Can you work these out from the model? Positions are in its coordinate system, mm. A direction names the side the tool comes from. Round coordinates to 2 decimals unless told otherwise and drop trailing zeros. Order: outer loops, then holes, each group sorted by start corner. A loop starts at its lowest first (then second) coordinate and runs counter-clockwise, first axis right, second up.
Autodesk Inventor part; units mm, degrees
ref_plane "YZ Plane" through (0, 0, 0) normal (1, 0, 0) x (0, 1, 0)
ref_plane "XZ Plane" through (0, 0, 0) normal (0, 1, 0) x (-1, 0, 0)
ref_plane "XY Plane" through (0, 0, 0) normal (0, 0, 1) x (1, 0, 0)
sketch "Sketch1" plane through (0, 0, 0) normal (0, 1, 0) x (-1, 0, 0)
  line L0 (-20, 12.5) -> (20, 12.5)
  line L1 (20, 12.5) -> (20, -12.5)
  line L2 (20, -12.5) -> (-20, -12.5)
  line L3 (-20, -12.5) -> (-20, 12.5)
  line L4 (-20, 12.5) -> (20, -12.5) construction
  line L5 (20, 12.5) -> (-20, -12.5) construction
  circle A0 centre (-4, 8.75) radius 2.25
  circle A1 centre (-4.5, -8.75) radius 2.25
  point P0 (0, 0)
  dimension "d0" = 40
  dimension "d1" = 25
  dimension "d49" = 4.5
  dimension "d50" = 4.5
extrude "Extrusion1" add sketch "Sketch1" along normal blind 3 contours L0 L1 L2 L3 | A0 | A1
sketch "Sketch3" plane through (-20, 0, -12.5) normal (-1, 0, 0) x (0, 0, 1)
  line L0 (0, 0) -> (25, 0)
  line L1 (0, 0) -> (25, 0)
  line L2 (25, 0) -> (25, 22)
  line L3 (25, 22) -> (0, 22)
  line L4 (0, 22) -> (0, 0)
  point P0 (12.5, 0)
  dimension "d14" = 22
extrude "Extrusion4" add sketch "Sketch3" along normal blind 9
sketch "Sketch4" plane through (-20, 22, 12.5) normal (0, 1, 0) x (1, 0, 0)
  line L0 (-4.7075, 24) -> (-1.5075, 24)
  line L1 (-1.5075, 24) -> (-1.5075, 1)
  line L2 (-1.5075, 1) -> (-4.7075, 1)
  line L3 (-4.7075, 1) -> (-4.7075, 24)
  point P0 (20, 12.5)
  dimension "d17" = 3.2
  dimension "d18" = 23
extrude "Extrusion5" cut sketch "Sketch4" against normal blind 21
sketch "Sketch6" plane through (-21.5075, 22, -11.5) normal (-1, 0, 0) x (0, 0, 1)
  line L0 (0, 0) -> (23, 0)
  line L1 (0, 0) -> (23, 0)
  line L2 (23, 0) -> (23, -3)
  line L3 (23, -3) -> (0, -3)
  line L4 (0, -3) -> (0, 0)
  point P0 (11.5, -22)
  dimension "d26" = 3
extrude "Extrusion7" cut sketch "Sketch6" against normal blind 3
sketch "Sketch5" plane through (-29, 0, -12.5) normal (-1, 0, 0) x (0, 0, 1)
  line L0 (20, 18.5) -> (20, 3.5)
  line L1 (20, 3.5) -> (5, 3.5)
  line L2 (5, 3.5) -> (5, 18.5)
  line L3 (5, 18.5) -> (20, 18.5)
  point P0 (12.5, 0)
  dimension "d21" = 15
  dimension "d22" = 15
extrude "Extrusion6" cut sketch "Sketch5" against normal blind 7
sketch "Sketch7" plane through (-29, 0, -12.5) normal (-1, 0, 0) x (0, 0, 1)
  line L0 (20, 3.5) -> (5, 3.5)
  line L1 (5, 3.5) -> (2, 3.5)
  line L2 (2, 3.5) -> (2, 22.5)
  line L3 (2, 22.5) -> (5, 22.5)
  line L4 (5, 22.5) -> (5, 3.5)
  line L5 (5, 22.5) -> (20, 22.5)
  line L6 (20, 22.5) -> (20, 18.5)
  line L7 (20, 18.5) -> (5, 18.5)
  line L8 (5, 18.5) -> (5, 22.5)
  line L9 (20, 3.5) -> (20, 22.5)
  line L10 (20, 22.5) -> (23, 22.5)
  line L11 (23, 22.5) -> (23, 3.5)
  line L12 (23, 3.5) -> (20, 3.5)
  line L13 (25, 0) -> (25, 22)
  point P0 (12.5, 0)
  dimension "d29" = 3
  dimension "d30" = 19
  dimension "d31" = 15
  dimension "d32" = 3
extrude "Extrusion8" add sketch "Sketch7" along normal blind 1 contours L1 L2 L3 L4
extrude "Extrusion9" add sketch "Sketch7" along normal blind 22 contours L9 L6 L10 L11 L12 | L7 L4 L5 L6
extrude "Extrusion10" add sketch "Sketch7" along normal blind 22 contours L1 L2 L3 L4
sketch "Sketch8" plane through (20, 0, 12.5) normal (0, 0, 1) x (1, 0, 0)
  line L0 (-40, 22) -> (-49, 22)
  line L1 (-49, 22) -> (-40, 22)
  line L2 (-40, 22) -> (-40, 0)
  line L3 (-40, 0) -> (-49, 0)
  line L4 (-49, 0) -> (-49, 22)
  point P0 (-20, 0)
extrude "Extrusion11" add sketch "Sketch8" along normal blind 2
sketch "Sketch9" plane through (20, 0, -12.5) normal (0, 0, -1) x (-1, 0, 0)
  line L0 (40, 22) -> (44.7075, 22)
  line L1 (49, 22) -> (40, 22)
  line L2 (40, 22) -> (40, 0)
  line L3 (40, 0) -> (49, 0)
  line L4 (49, 0) -> (49, 22)
  point P0 (20, 0)
extrude "Extrusion12" add sketch "Sketch9" along normal blind 2
sketch "Sketch10" plane through (-20, 0, -12.5) normal (1, 0, 0) x (0, 0, -1)
  line L0 (-27, 0) -> (-27, 22)
  line L1 (2, 22) -> (2, 0)
  line L2 (-27, 22) -> (2, 22)
  line L3 (2, 22) -> (2, 0)
  line L4 (2, 0) -> (-27, 0)
  line L5 (-27, 0) -> (-27, 22)
  point P0 (-12.5, 0)
extrude "Extrusion13" add sketch "Sketch10" along normal blind 2
sketch "Sketch11" plane through (-20, 0, -12.5) normal (-1, 0, 0) x (0, 0, 1)
  line L0 (1, 22) -> (1, 19)
  line L1 (1, 22) -> (24, 22)
  line L2 (1, 19) -> (1, 22)
  line L3 (1, 22) -> (24, 22)
  line L4 (24, 22) -> (24, 19)
  line L5 (24, 19) -> (1, 19)
  point P0 (12.5, 0)
extrude "Extrusion14" cut sketch "Sketch11" against normal blind 2
extrude "Extrusion15" cut sketch "Sketch1" along normal blind 3 contours A0 | A1
fillet "Fillet2" radius 3 2 edges at (-40, 22.5, 10.5) (-40, 22.5, -10.5)
sketch "Sketch12" plane through (20, 0, -12.5) normal (0, 0, -1) x (-1, 0, 0)
  line L0 (0, 3) -> (38, 3)
  line L1 (0, 3) -> (10, 3)
  line L2 (10, 3) -> (10, 0)
  line L3 (10, 0) -> (0, 0)
  line L4 (0, 0) -> (0, 3)
  point P0 (20, 0)
  dimension "d54" = 10
extrude "Extrusion16" cut sketch "Sketch12" against normal blind 25
properties part number "rgb-mount-group2"
(1) I want a section at B-B, the plane x = 4. List the corners of the cut face in (y, z) for me, plus the area to 3 significant figures.
(2) I want a section at C-C, the plane y = 6.25. List the corners of the cut face in (x, z) for me.
(3) On a 3-axis mill with a long thin cutter (end or side, diameter ignored), from which of +Z, -Z, +X, -X, +Y, -Y can I reach the whole of each face in a straight line? I mean faces 1 (the face through (-38, 11, -7.5)), 2 (the face through (-26, 22, 0)), 3 (the face through (-20, 19, 0)), 4 (the face through (-40, 12, 10.5)), 5 (the face through (-39.85, 21.64, 9.6)). Say none if no direction works.
(4) I'm going to push flat-ended pins straight in: pin 1 Ø4.5 at (x, y) = (-43.5, 10.5) entering from -Z; pin 2 Ø8 at (x, z) = (-40, 6.5) entering from -Y; pin 3 Ø3 at (x, z) = (-19.5, 1.5) entering from +Y; pin 4 Ø4.5 at (x, z) = (-27, -1.5) entering from +Y. Where does each tip first touch, or does it pass through?
(5) Please list where these lines run through material, in increasing order: probe 1 along Z at (x, y) = (-27.5, 7); probe 2 along X at (y, z) = (3.25, 6.75); probe 3 along Z at (x, y) = (4, 2.05).
(6) I want a section at A-A, the plane z = -2.25. List the corners of the cut face in (x, y) for me.
(7) I want a section at D-D, the plane x = -6.5. List the corners of the cut face in (y, z) for me, plus the area to 3 significant figures.
(8) If we mould it in two halves opening along Z, with no side actions, what happens to faces 6 (the face through (-40, 11, -10.5)), 7 (the face through (-27, 3.5, 0)), 8 (the face through (-51, 19, 0))? For each: pulls with the +Z half, pulls with the -Z half, needs draft (parallel to the pull), parting line crosses it, or undercut.
Ans:
1. outline: (0, -12.5) - (3, -12.5) - (3, -10.94) - (0, -10.94) - close; (0, -6.56) - (3, -6.56) - (3, 6.5) - (0, 6.5) - close; (0, 11) - (3, 11) - (3, 12.5) - (0, 12.5) - close
1. area: 48.3 mm2
2. outline: (-51, -10.5) - (-29, -10.5) - (-29, -14.5) - (-18, -14.5) - (-18, 14.5) - (-29, 14.5) - (-29, 10.5) - (-51, 10.5) - (-51, 7.5) - (-24.71, 7.5) - (-24.71, 11.5) - (-21.51, 11.5) - (-21.51, -11.5) - (-24.71, -11.5) - (-24.71, -7.5) - (-51, -7.5) - close
3. face 1: -X
3. face 2: +Z, -Z, +X, +Y
3. face 3: +X, +Y
3. face 4: +Z, -X, +Y, -Y
3. face 5: +Z, -X, +Y
4. pin 1: stops at z = -10.5
4. pin 2: stops at y = 3.5
4. pin 3: stops at y = 19
4. pin 4: stops at y = 22.5
5. probe 1: z = -14.5 to -7.5, 7.5 to 14.5
5. probe 2: x = -29 to -24.71, -21.51 to -18
5. probe 3: z = -12.5 to -10.94, -6.56 to 6.5, 11 to 12.5
6. outline: (-51, 18.5) - (-24.71, 18.5) - (-24.71, 22) - (-29, 22) - (-29, 22.5) - (-51, 22.5) - close; (-29, 0) - (10, 0) - (10, 3) - (-18, 3) - (-18, 19) - (-21.51, 19) - (-21.51, 1) - (-24.71, 1) - (-24.71, 3.5) - (-29, 3.5) - close
7. outline: (0, -12.5) - (3, -12.5) - (3, 12.5) - (0, 12.5) - close
7. area: 75.0 mm2
8. face 6: pulls with the -Z half
8. face 7: undercut
8. face 8: needs draft
